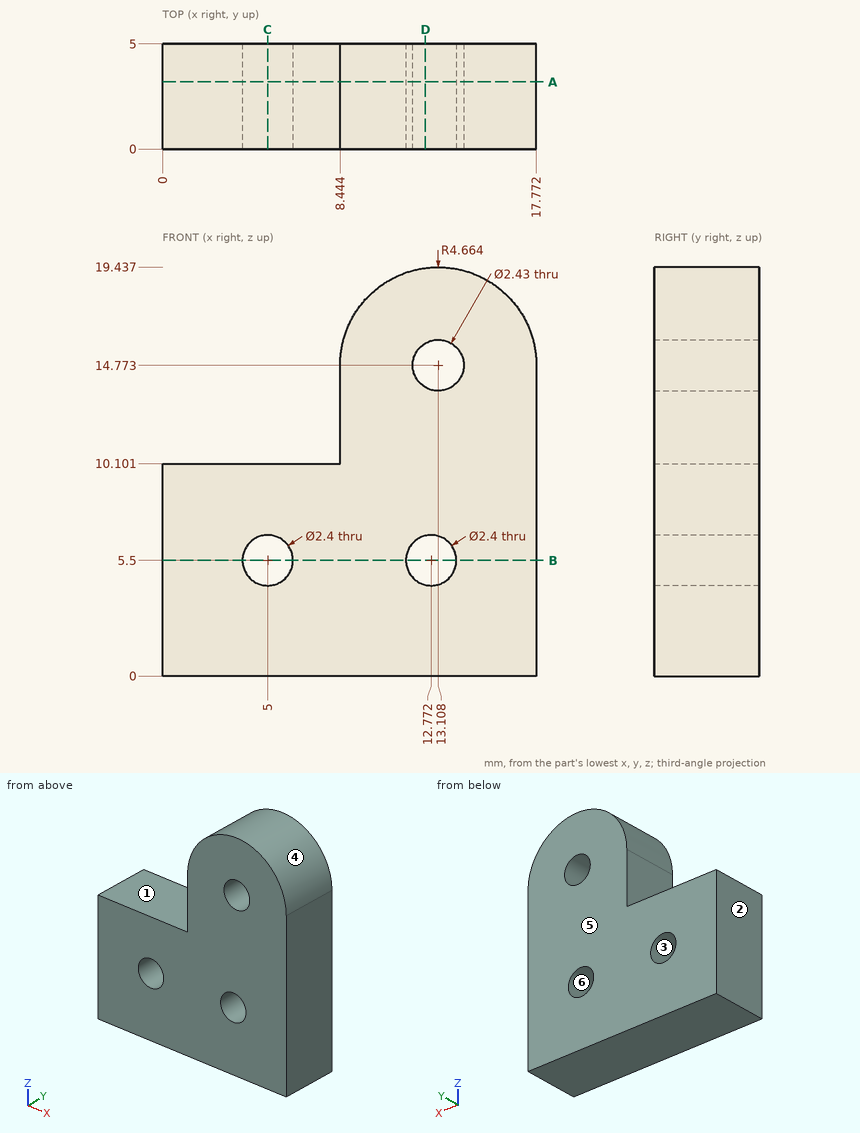
For this review, use the dimensioned drawing (mm, ordinates from the lowest corner) and the shaded views. A direction names the side the tool comes from. Coordinates: 2 decimals unless noted, no trailing zeros. Loops run counter-clockwise (first coordinate to the right, second up) from the corner with the lowest first, then second, coordinate; pieces in that order, holes last. Notation, with made-up numbers: M 86,87 L 119,87 A24 cw 119,107 Z; hole C 44,64 d9. An arc over 180 degrees is marked long. Answer as CSV lines item,"result".
Item 1: Add section D-D on x = 12.5. State the section outline as (y, z) points (1 decimal).
Answer list:
outline,"M 0,0 L 5,0 L 5,4.3 L 0,4.3 Z; M 0,6.7 L 5,6.7 L 5,13.7 L 0,13.7 Z; M 0,15.8 L 5,15.8 L 5,19.4 L 0,19.4 Z"
Item 2: Add section C-C on x = 5. State the section outline as (y, z) points, plus the area to 3 significant figures.
Answer list:
outline,"M 0,0 L 5,0 L 5,4.3 L 0,4.3 Z; M 0,6.7 L 5,6.7 L 5,10.1 L 0,10.1 Z"
area,"38.5 mm²"
Item 3: For probe 1 along X at (y, z) = (3.7, 5.5); probe 2 along Z at (x, y) = (5, 1.75); probe 3 along Z at (x, y) = (13.5, 3.2) (1 decimal), list the stretches that pass through material, from the lowest coordinate up.
Answer list:
probe 1,"0 to 3.8, 6.2 to 11.57, 13.97 to 17.77"
probe 2,"0 to 4.3, 6.7 to 10.1"
probe 3,"0 to 4.5, 6.5 to 13.6, 15.9 to 19.4"
Item 4: Machinability: for the marked faces 1 and 2, which of the approach directions +Z, -Z, +X, -X, +Y, -Y give a long, thin tool a straight path to every point of the face, cutting with its end or side? Answer none if there is none.
Answer list:
face 1,"+Z, -X, +Y, -Y"
face 2,"+Z, -Z, -X, +Y, -Y"
Item 5: The part is to be moulded in two halves that separate along Z. For the marked faces 3, 4, 5 and 6, say which applies: pulls with the +Z half, pulls with the -Z half, needs draft (parallel to the pull), parting line crosses it, or undercut.
Answer list:
face 3,"undercut"
face 4,"pulls with the +Z half"
face 5,"needs draft"
face 6,"undercut"
Item 6: For P1, Ø1.4, axis at y = 2.5, z = 13, coming from the -X side; P2, Ø1, axis at y = 4.5, z = 15.5, coming from the -X side; P3, Ø1, axis at x = 5.5, y = 2.5, coming from the +Z side; P4, Ø1.9, axis at x = 12.77, z = 5.5, coming from the -Y side, all flat-tipped, find the tip position at first contact; note any pin that passes through.
Answer list:
P1,"x = 8.44"
P2,"x = 8.45"
P3,"z = 10.1"
P4,"through"
Item 7: Add section A-A on y = 3.2. State the section outline as (x, z) points (1 decimal).
Answer list:
outline,"M 0,0 L 17.8,0 L 17.8,14.8 A4.7 ccw 8.4,14.8 L 8.4,10.1 L 0,10.1 Z; hole C 5,5.5 d2.4; hole C 12.8,5.5 d2.4; hole C 13.1,14.8 d2.4"
Item 8: Add section B-B on z = 5.5. State the section outline as (x, y) points.
Answer list:
outline,"M 0,0 L 3.8,0 L 3.8,5 L 0,5 Z; M 6.2,0 L 11.57,0 L 11.57,5 L 6.2,5 Z; M 13.97,0 L 17.77,0 L 17.77,5 L 13.97,5 Z"
